Design review of the part shown in the three views and the two pictorial views. Dimensions are in mm from the part's minimum x, y and z. Coordinates: 2 decimals unless noted, no trailing zeros. Loops run counter-clockwise (first coordinate to the right, second up) from the corner with the lowest first, then second, coordinate; pieces in that order, holes last. Notation, with made-up numbers: (-40, 60.25) -> (12, 60.25) arc R11 cw to (12, 80.25) -> close; hole circle Ø11 at (56.5, 67). An arc over 180 degrees is marked (long way). Use CSV: the item, a comma, the result in double quotes.
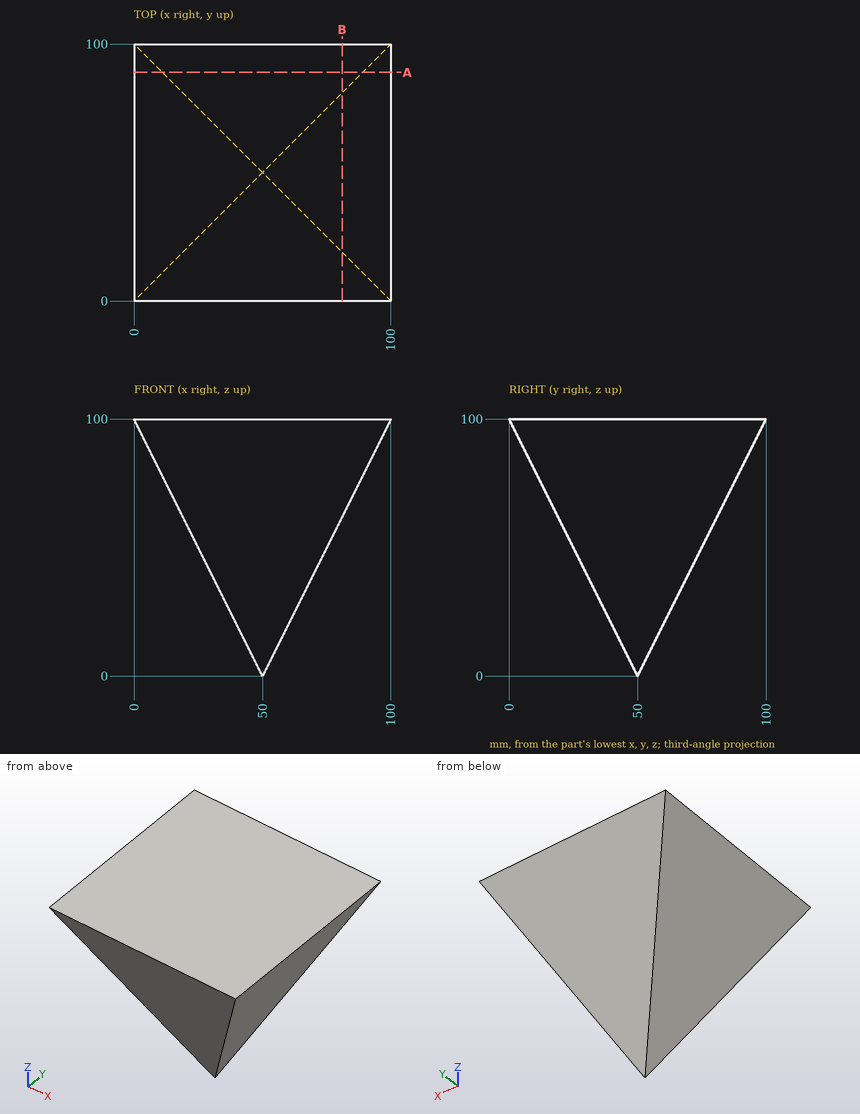
Item 1: To check wall thickness, follow line 1 along X through (y, z) = (36.5, 75); line 2 along X through (y, z) = (48, 7); line 3 along Z through (x, y) = (8, 17.5). State the ranges of each line that lie inside material, in increasing order.
Checked values:
line 1,"12.5 to 87.5"
line 2,"46.5 to 53.5"
line 3,"84 to 100"
Item 2: Clearance check with flat-ended pins moving along their axes: pin 1 (12 mm diameter, centred on y = 43.5, z = 79, fed in from -X); pin 2 (10 mm diameter, centred on y = 24.5, z = 52, fed in from -X); pin 3 (10 mm diameter, centred on x = 25, z = 71, fed in from -Y). State where each tip first meets the part, or that it passes through.
Checked values:
pin 1,"x = 7.5"
pin 2,"x = 21.5"
pin 3,"y = 12"
Item 3: Add section A-A (y = 89). Give the boundary of the cut face in (x, z).
Checked values:
outline,"(0, 100) -> (11, 78) -> (89, 78) -> (100, 100) -> close"
Item 4: Add section B-B (x = 81). Give the boundary of the cut face in (y, z).
Checked values:
outline,"(0, 100) -> (19, 62) -> (81, 62) -> (100, 100) -> close"
